For this review, take the finished solid that the model builds, in its own axes (mm). Face numbers are marked on the shaded views. A direction names the side the tool comes from. Coordinates: 2 decimals unless noted, no trailing zeros. Loops run counter-clockwise (first coordinate to the right, second up) from the corner with the lowest first, then second, coordinate; pieces in that order, holes last. Notation, with made-up numbers: M 78,32 L 93,32 A24 ccw 93,62 Z; hole C 37,49.25 d9. An arc over 180 degrees is marked long. Answer as a JSON object with one key per item and string values. Group by question number.
Item 1: Mouldability with a two-part tool opening along X and no side actions: class the marked faces 1, 2, 3 and 4 as +X half, -X half, draft (parallel to the pull), parting line (faces both ways), or undercut.
Item 2: Add section D-D (z = 10.75). State the section outline as (x, y) points, then the cut area to 3 significant figures.
Item 3: Add section A-A (x = -12.5). State the section outline as (y, z) points.
Item 4: Add section C-C (y = 49.5). State the section outline as (x, z) points, then the cut area to 3 significant figures.
Item 5: Add section B-B (z = 7.25). State the section outline as (x, y) points.
Item 6: Tool access review of the marked faces 5 and 6: name each direction out of +Z, -Z, +X, -X, +Y, -Y from which nothing blocks a thin tool from reaching the whole face with its end or side.
Item 7: Wall thickness on L1, parallel to X at y = 42.5, z = 6.5; L2, parallel to X at y = 55.25, z = 3; L3, parallel to Z at x = -7.5, y = 54: over which ranges is each line inside the solid? List them lowest first. Write a range as from..to.
Item 8: Insertion check: pin 1 (5.5 mm diameter, centred on x = -2.49, z = 6.5, fed in from +Y); pin 2 (5 mm diameter, centred on x = -15.5, y = 53, fed in from +Z). Each pin has a flat end and moves straight along its axis. Give the tip position at first contact, or say it passes through.
from build123d import *

# Parameters (mm, degrees)
SKETCH1_W            = 42
SKETCH1_H            = 18.183578202
BOSS_EXTRUDE1_DEPTH  = 1.5
SKETCH2_W            = 42
SKETCH2_H            = 2
BOSS_EXTRUDE2_DEPTH  = 10
BOSS_EXTRUDE4_DEPTH  = 1.5
BOSS_EXTRUDE5_START  = -42
BOSS_EXTRUDE5_DEPTH  = 1.5
M3_CLEARANCE_HOLE2_D = 3.4
FILLET4_R            = 0.2


with BuildPart() as part:
    # Sketch1 → Boss-Extrude1 (new body)
    with BuildSketch(Plane.XY):
        with Locations((-17.985553167, 50.952165471)):
            Rectangle(SKETCH1_W, SKETCH1_H)
        Polygon((-27.135553167, 52.575255776), (-27.135553167, 53.075255776), (-27.985553167, 53.075255776), (-27.985553167, 54.675255776), (-31.985553167, 54.675255776), (-31.985553167, 53.075255776), (-32.835553167, 53.075255776), (-32.835553167, 52.575255776), (-34.985553167, 52.575255776), (-34.985553167, 48.425255776), (-32.835553167, 48.425255776), (-32.835553167, 47.925255776), (-27.135553167, 47.925255776), (-27.135553167, 48.425255776), (-24.985553167, 48.425255776), (-24.985553167, 52.575255776), align=None, mode=Mode.SUBTRACT)
        Polygon((-14.135553167, 52.575255776), (-14.135553167, 53.075255776), (-14.985553167, 53.075255776), (-14.985553167, 54.675255776), (-18.985553167, 54.675255776), (-18.985553167, 53.075255776), (-19.835553167, 53.075255776), (-19.835553167, 52.575255776), (-21.985553167, 52.575255776), (-21.985553167, 48.425255776), (-19.835553167, 48.425255776), (-19.835553167, 47.925255776), (-14.135553167, 47.925255776), (-14.135553167, 48.425255776), (-11.985553167, 48.425255776), (-11.985553167, 52.575255776), align=None, mode=Mode.SUBTRACT)
        Polygon((-1.135553167, 52.575255776), (-1.135553167, 53.075255776), (-1.985553167, 53.075255776), (-1.985553167, 54.675255776), (-5.985553167, 54.675255776), (-5.985553167, 53.075255776), (-6.835553167, 53.075255776), (-6.835553167, 52.575255776), (-8.985553167, 52.575255776), (-8.985553167, 48.425255776), (-6.835553167, 48.425255776), (-6.835553167, 47.925255776), (-1.135553167, 47.925255776), (-1.135553167, 48.425255776), (1.014446833, 48.425255776), (1.014446833, 52.575255776), align=None, mode=Mode.SUBTRACT)
    extrude(amount=BOSS_EXTRUDE1_DEPTH)

    # Sketch2 → Boss-Extrude2 (add)
    with BuildSketch(Plane.XY.offset(1.5)):
        with Locations((-17.985553167, 42.86037637)):
            Rectangle(SKETCH2_W, SKETCH2_H)
    extrude(amount=BOSS_EXTRUDE2_DEPTH)

    # Sketch7 → Boss-Extrude4 (add)
    with BuildSketch(Plane.ZY.offset(38.985553167)):
        Polygon((1.5, 60.043954572), (0, 60.043954572), (0, 41.86037637), (11.5, 41.86037637), (11.5, 43.86037637), (1.5, 43.86037637), align=None)
        Polygon((11.5, 43.86037637), (1.5, 60.043954572), (1.5, 43.86037637), align=None)
    extrude(amount=BOSS_EXTRUDE4_DEPTH)

    # Sketch7_3 → Boss-Extrude5 (add)
    with BuildSketch(Plane.ZY.offset(38.985553167).offset(BOSS_EXTRUDE5_START)):
        Polygon((11.5, 43.86037637), (1.5, 60.043954572), (1.5, 43.86037637), align=None)
        Polygon((1.5, 60.043954572), (0, 60.043954572), (0, 41.86037637), (11.5, 41.86037637), (11.5, 43.86037637), (1.5, 43.86037637), align=None)
    extrude(amount=-BOSS_EXTRUDE5_DEPTH)

    # M3 Clearance Hole2 (through all)
    with Locations(Plane(origin=(0, 43.86037637, 0), x_dir=(1, 0, 0), z_dir=(0, 1, 0))):
        with Locations((-33.485553167, -6.5), (-2.485553167, -6.5)):
            Hole(M3_CLEARANCE_HOLE2_D / 2)

    # Fillet4
    fillet4_edges = [part.edges().sort_by_distance(p)[0] for p in [
        (-8.985553167, 50.500255776, 1.5),
        (1.014446833, 50.500255776, 1.5),
        (-34.985553167, 50.500255776, 1.5),
        (-24.985553167, 50.500255776, 1.5),
        (-21.985553167, 50.500255776, 1.5),
        (-11.985553167, 50.500255776, 1.5),
    ]]
    fillet(fillet4_edges, radius=FILLET4_R)


solid = part.part
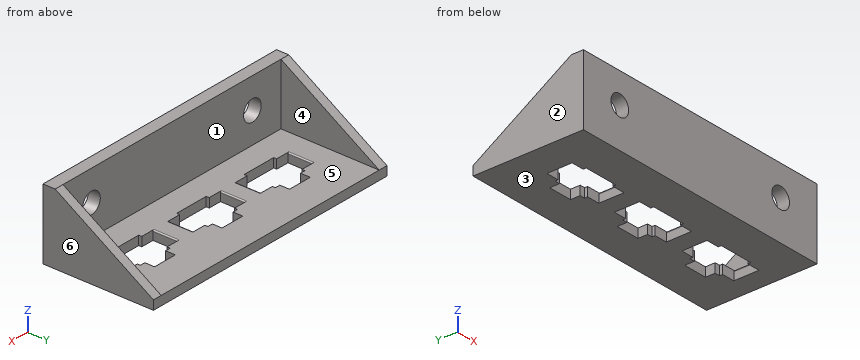
From the geometry:
{
 "1": {"face 1": "undercut", "face 2": "-X half", "face 3": "draft", "face 4": "undercut"},
 "2": {"outline": "M -40.49,41.86 L 4.51,41.86 L 4.51,45.07 L 3.01,45.07 L 3.01,43.86 L -38.99,43.86 L -38.99,45.07 L -40.49,45.07 Z", "area": "93.6 mm²"},
 "3": {"outline": "M 41.86,0 L 48.43,0 L 48.43,1.5 L 43.86,1.5 L 43.86,11.5 L 41.86,11.5 Z; M 52.58,0 L 60.04,0 L 60.04,1.5 L 52.58,1.5 Z"},
 "4": {"outline": "M -40.49,0 L -34.99,0 L -34.99,1.3 A0.2 ccw -35.19,1.5 L -38.99,1.5 L -38.99,8.02 L -40.49,8.02 Z; M -24.99,0 L -21.99,0 L -21.99,1.3 A0.2 ccw -22.19,1.5 L -24.79,1.5 A0.2 ccw -24.99,1.3 Z; M -11.99,0 L -8.99,0 L -8.99,1.3 A0.2 ccw -9.19,1.5 L -11.79,1.5 A0.2 ccw -11.99,1.3 Z; M 1.01,0 L 4.51,0 L 4.51,8.02 L 3.01,8.02 L 3.01,1.5 L 1.21,1.5 A0.2 ccw 1.01,1.3 Z", "area": "42.0 mm²"},
 "5": {"outline": "M -40.49,41.86 L -35.01,41.86 L -35.01,43.86 L -38.99,43.86 L -38.99,50.74 L -40.49,50.74 Z; M -31.96,41.86 L -4.01,41.86 L -4.01,43.86 L -31.96,43.86 Z; M -0.96,41.86 L 4.51,41.86 L 4.51,50.74 L 3.01,50.74 L 3.01,43.86 L -0.96,43.86 Z"},
 "6": {"face 5": "+Z, +Y", "face 6": "+Z, -Z, +X, +Y, -Y"},
 "7": {"L1": "x = -40.49..-35.19, -31.79..-4.19, -0.79..4.51", "L2": "x = -40.49..-38.99, 3.01..4.51", "L3": "z = 0..1.5"},
 "8": {"pin 1": "stops at y = 43.86", "pin 2": "stops at z = 1.5"}
}
